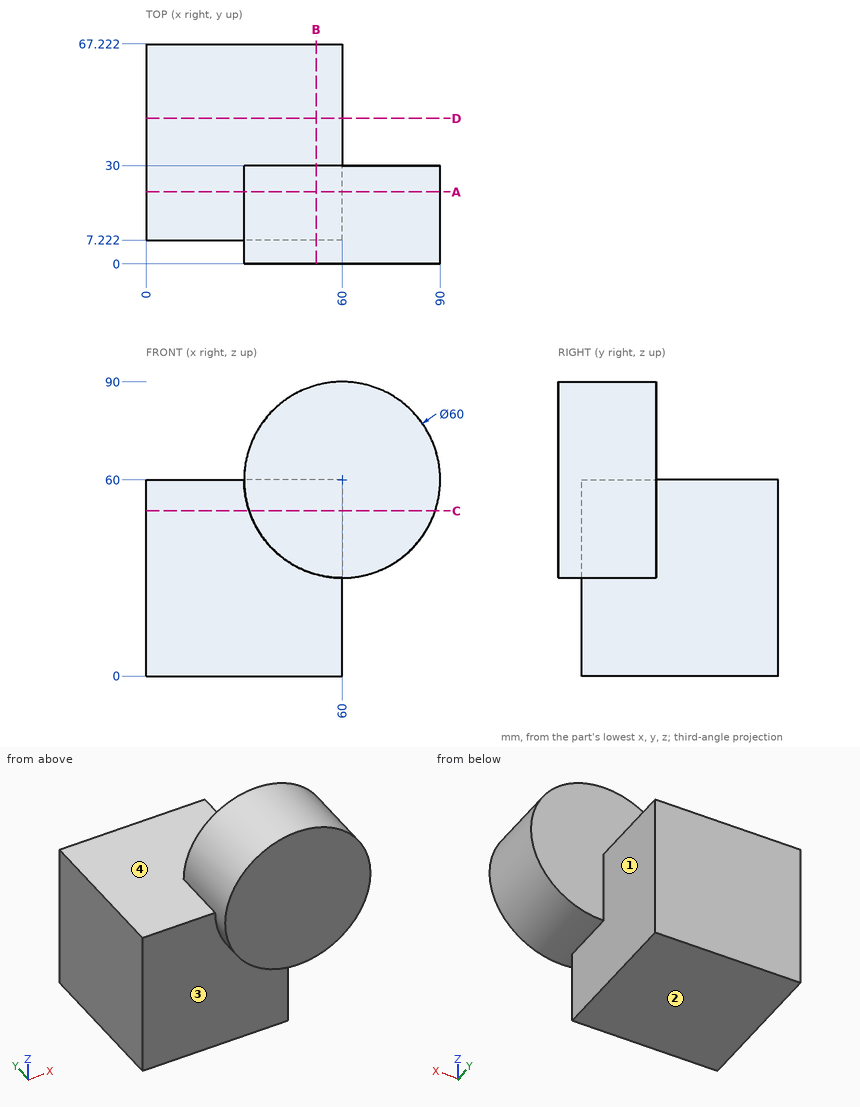
Geometry check sheet. Reference: drawing and pictorial views, mm from the part's lowest x, y, z. A direction names the side the tool comes from. Give positions to 0.01 mm unless a question says otherwise; leave off trailing zeros. Write each loop counter-clockwise with the first axis right and the second up, starting at its lowest first coordinate (ties: lowest second). Pieces come first, ordered by that corner, then holes. Notation, with made-up numbers: (72, -10) -> (119, -10) arc R23 cw to (119, 4) -> close; hole circle Ø11 at (-19, 58). An arc over 180 degrees is marked (long way). One line per question, with ' | ' between items.
Item 1: Sectioned sample at B-B, the plane x = 52. Record the boundary of the cut face in (y, z), plus the area to 3 significant figures.
Determined:
outline: (0, 31.09) -> (7.22, 31.09) -> (7.22, 0) -> (67.22, 0) -> (67.22, 60) -> (30, 60) -> (30, 88.91) -> (0, 88.91) -> close | area: 4,680 mm^2
Item 2: Sectioned sample at A-A, the plane y = 22. Record the boundary of the cut face in (x, z), plus the area to 3 significant figures.
Determined:
outline: (0, 0) -> (60, 0) -> (60, 30) arc R30 ccw (long way) to (30, 60) -> (0, 60) -> close | area: 5,720 mm^2
Item 3: Scan lines: line 1 along X through (y, z) = (38, 29.5); line 2 along Y through (x, z) = (62.5, 70.5). Record each from-to range of solid material in increasing order.
Determined:
line 1: 0 to 60 | line 2: 0 to 30
Item 4: Sectioned sample at D-D, the plane y = 44.5. Record the boundary of the cut face in (x, z), plus the area to 3 significant figures.
Determined:
outline: (0, 0) -> (60, 0) -> (60, 60) -> (0, 60) -> close | area: 3,600 mm^2
Item 5: Depth check by flat-ended pin: pin 1 (12 mm diameter, centred on y = 34, z = 35.5, fed in from +X) (1 decimal); pin 2 (1.5 mm diameter, centred on x = 70.5, z = 54.5, fed in from +Y); pin 3 (18 mm diameter, centred on x = 39, y = 27.5, fed in from +Z) (1 decimal). Enter the tip coordinate at first touch or a pass-through.
Determined:
pin 1: x = 82.3 | pin 2: y = 30 | pin 3: z = 87.5
Item 6: Access from +Z, -Z, +X, -X, +Y, -Y to the whole of each face (thin tool, end or side, straight path). Record for the marked faces 1, 2, 3 and 4.
Determined:
face 1: -Z, +X, +Y | face 2: -Z, +X, -X, +Y, -Y | face 3: -Z, -X, -Y | face 4: +Z, -X, +Y
Item 7: Sectioned sample at C-C, the plane z = 50.5. Record the boundary of the cut face in (x, y).
Determined:
outline: (0, 7.22) -> (31.54, 7.22) -> (31.54, 0) -> (88.46, 0) -> (88.46, 30) -> (60, 30) -> (60, 67.22) -> (0, 67.22) -> close
